Verification items for the finished model (mm, model axes). Face numbers are marked on the shaded views. A direction names the side the tool comes from. Coordinates: 2 decimals unless noted, no trailing zeros. Write each loop counter-clockwise with the first axis right and the second up, starting at its lowest first coordinate (ties: lowest second). Pieces come first, ordered by that corner, then holes. Notation, with made-up numbers: M -2.75,79 L 3.25,79 A21 cw 3.25,115 Z; hole C 4,5.25 d2. An arc over 180 degrees is marked long. Answer in a Markdown table with one row per item.
from build123d import *

# Parameters (mm, degrees)
CROQUIS1_R              = 10
SALIENTE_EXTRUIR1_DEPTH = 16
CROQUIS2_R              = 2
CORTAR_EXTRUIR1_DEPTH   = 20
CORTAR_EXTRUIR2_DEPTH   = 3
CROQUIS5_R              = 1
CORTAR_EXTRUIR3_DEPTH   = 14.0000001


with BuildPart() as part:
    # Croquis1 → Saliente-Extruir1 (new body)
    with BuildSketch(Plane.XY):
        Circle(CROQUIS1_R)
        with BuildLine():
            Line((2.611340652, 3.03), (-2.611340652, 3.03))
            ThreePointArc((-2.611340652, 3.03), (0, -4), (2.611340652, 3.03))
        make_face(mode=Mode.SUBTRACT)
    extrude(amount=SALIENTE_EXTRUIR1_DEPTH)

    # Croquis2 → Cortar-Extruir1 (cut)
    with BuildSketch(Plane(origin=(0, 0, 0), x_dir=(1, 0, 0), z_dir=(0, 1, 0))):
        with Locations((0, -4)):
            Circle(CROQUIS2_R)
        with Locations((0, -10.5)):
            Circle(CROQUIS2_R)
    extrude(amount=CORTAR_EXTRUIR1_DEPTH, mode=Mode.SUBTRACT)

    # Croquis3 → Cortar-Extruir2 (cut)
    with BuildSketch(Plane(origin=(0, 0, 0), x_dir=(-1, 0, 0), z_dir=(0, 0, -1))):
        Polygon((-3.5, 5), (-4.25, 6.299038106), (-5.75, 6.299038106), (-6.5, 5), (-5.75, 3.700961894), (-4.25, 3.700961894), align=None)
        Polygon((6.499503191, 5.038602866), (5.716320533, 6.317909289), (4.216817342, 6.279306423), (3.500496809, 4.961397134), (4.283679467, 3.682090711), (5.783182658, 3.720693577), align=None)
        Polygon((6.499999707, -5.000936904), (5.750811237, -3.7014306), (4.250811529, -3.700493696), (3.500000293, -4.999063096), (4.249188763, -6.2985694), (5.749188471, -6.299506304), align=None)
        Polygon((-3.500204706, -4.975219447), (-4.271562941, -3.688748898), (-5.771358235, -3.713529451), (-6.499795294, -5.024780553), (-5.728437059, -6.311251102), (-4.228641765, -6.286470549), align=None)
    extrude(amount=-CORTAR_EXTRUIR2_DEPTH, mode=Mode.SUBTRACT)

    # Croquis5 → Cortar-Extruir3 (cut, through all)
    with BuildSketch(Plane(origin=(0, 0, 3), x_dir=(-1, 0, 0), z_dir=(0, 0, -1))):
        with Locations((-5, 5)):
            Circle(CROQUIS5_R)
        with Locations((5, 5)):
            Circle(CROQUIS5_R)
        with Locations((5.000811383, -4.999063096)):
            Circle(CROQUIS5_R)
        with Locations((-5, -4.999063096)):
            Circle(CROQUIS5_R)
    extrude(amount=-CORTAR_EXTRUIR3_DEPTH, mode=Mode.SUBTRACT)


solid = part.part
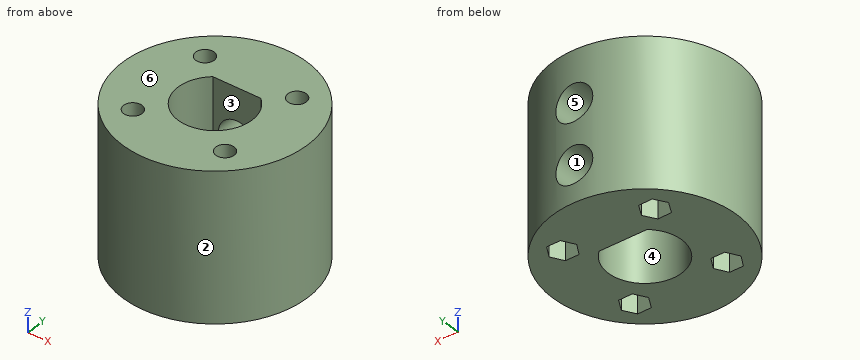
1) Tool access check on the marked faces 5 and 6. Record the directions out of +Z, -Z, +X, -X, +Y, -Y that give a thin tool (end or side, any length) a straight path to the whole face; none if there is none.
Response values:
| item | result |
|---|---|
| face 5 | +Y |
| face 6 | +Z, +X, -X, +Y, -Y |
2) Thickness scan on L1, parallel to X at y = -4.5, z = 15.25; L2, parallel to Y at x = -5, z = 11.5. Record the ranges inside material, lowest first. Write a range as [from, to].
Response values:
| item | result |
|---|---|
| L1 | x = [-8.93, -5.87], [-4.13, 4.13], [5.87, 8.93] |
| L2 | y = [-8.66, -6], [-4, 4], [6, 8.66] |
3) Sectioned sample at A-A (z = 1.5). Record the cut outline in (x, y), then the cut area to 3 significant figures.
Response values:
| item | result |
|---|---|
| outline | C 0,0 d20; hole M -6.5,-5 L -5.75,-6.3 L -4.25,-6.3 L -3.5,-5 L -4.25,-3.7 L -5.75,-3.7 Z; hole M -6.5,5.04 L -5.78,3.72 L -4.28,3.68 L -3.5,4.96 L -4.22,6.28 L -5.72,6.32 Z; hole M -2.61,3.03 A4 ccw long 2.61,3.03 Z; hole M 3.5,-4.98 L 4.23,-6.29 L 5.73,-6.31 L 6.5,-5.02 L 5.77,-3.71 L 4.27,-3.69 Z; hole M 3.5,5 L 4.25,3.7 L 5.75,3.7 L 6.5,5 L 5.75,6.3 L 4.25,6.3 Z |
| area | 244 mm² |
4) Release check for a two-part mould opening along Y. For the marked faces 1, 2, 3 and 4 record: +Y half, -Y half, draft (parallel to the pull), parting line (faces both ways), or undercut.
Response values:
| item | result |
|---|---|
| face 1 | draft |
| face 2 | parting line |
| face 3 | undercut |
| face 4 | undercut |
5) Sectioned sample at D-D (z = 4). Record the cut outline in (x, y).
Response values:
| item | result |
|---|---|
| outline | M -2.61,3.03 L -2,3.03 L -2,9.8 A10 ccw long 2,9.8 L 2,3.03 L 2.61,3.03 A4 cw long Z; hole C -5,-5 d2; hole C -5,5 d2; hole C 5,-5 d2; hole C 5,5 d2 |
6) Depth check by flat-ended pin: pin 1 (1.8 mm diameter, centred on x = 5, y = 5, fed in from +Z); pin 2 (1.6 mm diameter, centred on x = 4.5, z = 1, fed in from -Y); pin 3 (6 mm diameter, centred on x = 4, z = 12.5, fed in from -Y); pin 4 (4 mm diameter, centred on x = -6, z = 5.5, fed in from -Y). Enter the tip coordinate at first touch or a pass-through.
Response values:
| item | result |
|---|---|
| pin 1 | passes through |
| pin 2 | stops at y = -9.29 |
| pin 3 | stops at y = -9.95 |
| pin 4 | stops at y = -9.17 |
7) Sectioned sample at B-B (y = 0). Record the cut outline in (x, z), then the cut area to 3 significant figures.
Response values:
| item | result |
|---|---|
| outline | M -10,0 L -4,0 L -4,16 L -10,16 Z; M 4,0 L 10,0 L 10,16 L 4,16 Z |
| area | 192 mm² |
8) Sectioned sample at C-C (x = 0). Record the cut outline in (y, z), then the cut area to 3 significant figures.
Response values:
| item | result |
|---|---|
| outline | M -10,0 L -4,0 L -4,16 L -10,16 Z; M 3.03,0 L 10,0 L 10,2 L 3.03,2 Z; M 3.03,6 L 10,6 L 10,8.5 L 3.03,8.5 Z; M 3.03,12.5 L 10,12.5 L 10,16 L 3.03,16 Z |
| area | 152 mm² |
